from build123d import *

# Parameters (mm, degrees)
BOSS_EXTRU_1_DEPTH = 10
CONG_2_R           = 16
CONG_3_R           = 10
CONG_4_R           = 50


with BuildPart() as part:
    # Esquisse1 → Boss.-Extru.1 (new body)
    with BuildSketch(Plane.XY):
        Polygon((80, 171), (0, 171), (0, 191), (100, 191), (218, 291), (218, 141), (230, 141), (230, 110.169491525), (100, 0), (0, 0), (0, 20), (80, 20), align=None)
    extrude(amount=BOSS_EXTRU_1_DEPTH)

    # Congé2
    cong_2_edges = [part.edges().sort_by_distance(p)[0] for p in [
        (80, 20, 5),
        (80, 171, 5),
    ]]
    fillet(cong_2_edges, radius=CONG_2_R)

    # Congé3
    cong_3_edges = [part.edges().sort_by_distance(p)[0] for p in [
        (0, 191, 5),
        (0, 0, 5),
    ]]
    fillet(cong_3_edges, radius=CONG_3_R)

    # Congé4
    cong_4_edges = [part.edges().sort_by_distance(p)[0] for p in [
        (100, 191, 5),
        (230, 110.169491525, 5),
        (100, 0, 5),
    ]]
    fillet(cong_4_edges, radius=CONG_4_R)


solid = part.part
Source: CAD feature listing. Evaluate the final solid. Frame: model axes, mm. A direction names the side the tool comes from. Coordinates: 2 decimals unless noted, no trailing zeros. Loops run counter-clockwise (first coordinate to the right, second up) from the corner with the lowest first, then second, coordinate; pieces in that order, holes last. Notation, with made-up numbers: M -30.75,3.25 L -4.75,3.25 A16 cw -4.75,33.25 Z; hole C 21,31 d11. An arc over 180 degrees is marked long. Answer in a Markdown table with one row per item.
Q1. Set-up query: faces 1 (the flat face through (218, 217, 5)), 2 (the cylindrical face through (75.189, 166.437, 5.07)), 3 (the cylindrical face through (98.648, 193.973, 5.07)). Return all of +Z, -Z, +X, -X, +Y, -Y with unobstructed straight access to the full face (end or side cutting, diameter ignored); none if empty.
Answers below:
| item | result |
|---|---|
| face 1 | +Z, -Z, +X, +Y |
| face 2 | +Z, -Z, -X |
| face 3 | +Z, -Z, -X, +Y |
Q2. Section A-A on x = 28. Return the cut outline in (y, z).
Answers below:
| item | result |
|---|---|
| outline | M 0,0 L 20,0 L 20,10 L 0,10 Z; M 171,0 L 191,0 L 191,10 L 171,10 Z |
Q3. First-contact query: pin 1 (4 mm diameter, centred on y = 57.5, z = 3, fed in from -X); pin 2 (3 mm diameter, centred on x = 116.5, y = 190.5, fed in from -Z); pin 3 (3 mm diameter, centred on y = 187, z = 2.5, fed in from +X); pin 4 (5 mm diameter, centred on x = 134.5, z = 7.5, fed in from -Y). Flat tips, straight axial feed; report the tip coordinate or a pass-through.
Answers below:
| item | result |
|---|---|
| pin 1 | stops at x = 80 |
| pin 2 | stops at z = 0 |
| pin 3 | stops at x = 218 |
| pin 4 | stops at y = 27.12 |
Q4. Draft query along Y for faces 4 (the flat face through (32, 171, 5)), 5 (the flat face through (0, 176, 5)), 6 (the cylindrical face through (75.189, 24.563, 5.07)), 7 (the flat face through (224, 141, 5)). Return one class per face: pulls with the +Y half, pulls with the -Y half, needs draft (parallel to the pull), parting line crosses it, or undercut.
Answers below:
| item | result |
|---|---|
| face 4 | undercut |
| face 5 | needs draft |
| face 6 | undercut |
| face 7 | pulls with the +Y half |
Q5. Section C-C on y = 174.5. Return the cut outline in (x, z), plus the area to 3 significant figures.
Answers below:
| item | result |
|---|---|
| outline | M 0,0 L 218,0 L 218,10 L 0,10 Z |
| area | 2,180 mm^2 |
Q6. Section D-D on x = 72.5. Return the cut outline in (y, z).
Answers below:
| item | result |
|---|---|
| outline | M 0,0 L 22.44,0 L 22.44,10 L 0,10 Z; M 168.56,0 L 191,0 L 191,10 L 168.56,10 Z |
Q7. Section B-B on z = 2.75. Return the cut outline in (x, y), plus the area to 3 significant figures.
Answers below:
| item | result |
|---|---|
| outline | M 0,10 A10 ccw 10,0 L 81.66,0 A50 ccw 113.99,11.86 L 212.33,95.19 A50 ccw 230,133.34 L 230,141 L 218,141 L 218,291 L 113.99,202.86 A50 cw 81.66,191 L 10,191 A10 ccw 0,181 L 0,171 L 64,171 A16 cw 80,155 L 80,36 A16 cw 64,20 L 0,20 Z |
| area | 30,000 mm^2 |
Q8. Ray query, probe 1 along Y at (x, z) = (33, 2.75); probe 2 along X at (y, z) = (152.5, 5.5); probe 3 along X at (y, z) = (179.5, 2.5). Return the intervals inside material, ascending. Write a range as from..to.
Answers below:
| item | result |
|---|---|
| probe 1 | y = 0..20, 171..191 |
| probe 2 | x = 80..218 |
| probe 3 | x = 0..218 |
